```python
from build123d import *

# Parameters (mm, degrees)
SKETCH1_R           = 14
SKETCH1_R_2         = 8
BOSS_EXTRUDE1_DEPTH = 3.5
CUT_EXTRUDE1_START  = -0.5
SKETCH2_R           = 13
SKETCH2_R_2         = 9
CUT_EXTRUDE1_DEPTH  = 22.5


with BuildPart() as part:
    # Sketch1 → Boss-Extrude1 (new, symmetric)
    with BuildSketch(Plane.XY):
        Circle(SKETCH1_R)
        Circle(SKETCH1_R_2, mode=Mode.SUBTRACT)
    extrude(amount=BOSS_EXTRUDE1_DEPTH, both=True)

    # Sketch2 → Cut-Extrude1 (cut)
    with BuildSketch(Plane.XY.offset(3.5).offset(CUT_EXTRUDE1_START)):
        with Locations(Location((0, 0, 0), (0, 0, 180))):
            Circle(SKETCH2_R)
        with Locations(Location((0, 0, 0), (0, 0, 180))):
            Circle(SKETCH2_R_2, mode=Mode.SUBTRACT)
    cut_extrude1 = extrude(amount=CUT_EXTRUDE1_DEPTH, mode=Mode.SUBTRACT)

    # Mirror1: Cut-Extrude1 across plane
    add(cut_extrude1.mirror(Plane.XY), mode=Mode.SUBTRACT)

    # Mirror1 at the second plane: Cut-Extrude1 across plane
    add(cut_extrude1.mirror(Plane(origin=(0, 0, 0), x_dir=(0, 0, 1), z_dir=(1, 0, 0))), mode=Mode.SUBTRACT)


solid = part.part
```
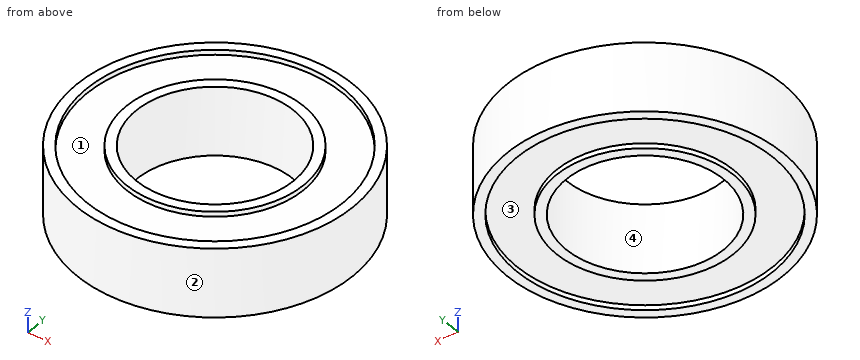
Source: CAD feature listing. Evaluate the final solid. Frame: model axes, mm. Face numbers are marked on the shaded views. A direction names the side the tool comes from. Round coordinates to 2 decimals unless told otherwise and drop trailing zeros. Loops run counter-clockwise (first coordinate to the right, second up) from the corner with the lowest first, then second, coordinate; pieces in that order, holes last.
1. Section query C-C on y = -12.25. Output: boundary loops of the cut face in (x, z), and give its area (3 significant figures).
2. Section query A-A on y = 0. Output: boundary loops of the cut face in (x, z), and give its area (3 significant figures).
3. Section query D-D on z = 1.25. Output: boundary loops of the cut face in (x, y), and give its area (3 significant figures).
4. Mould query, pull axis X, two halves, no side actions, for the marked faces 1 and 2. Classes: released by +X, released by -X, zero draft, split by the parting line, or undercut.
5. Contact query for flat-ended pins moving along their axis: pin 1 (3 mm diameter, centred on y = -8, z = 2, fed in from +X); pin 2 (2 mm diameter, centred on y = -2, z = -1.5, fed in from -X); pin 3 (4 mm diameter, centred on y = 7, z = -2.5, fed in from -X). Output: stop coordinate, or through.
6. Ray query, L1, parallel to Y at x = 0, z = -3.2; L2, parallel to Y at x = 0, z = 1.25; L3, parallel to X at y = -2.75, z = -0.5. Return the intervals inside material, ascending.
7. Access query for the marked faces 3 and 4. Directions: +Z, -Z, +X, -X, +Y, -Y. A direction counts if a zero-diameter tool reaches every point of the face in a straight line with its end or side. Return the directions, or none.
Answers below:
1. outline: (-6.78, -3.5) - (-4.35, -3.5) - (-4.35, -3) - (4.35, -3) - (4.35, -3.5) - (6.78, -3.5) - (6.78, 3.5) - (4.35, 3.5) - (4.35, 3) - (-4.35, 3) - (-4.35, 3.5) - (-6.78, 3.5) - close
1. area: 86.2 mm2
2. outline: (-14, -3.5) - (-13, -3.5) - (-13, -3) - (-9, -3) - (-9, -3.5) - (-8, -3.5) - (-8, 3.5) - (-9, 3.5) - (-9, 3) - (-13, 3) - (-13, 3.5) - (-14, 3.5) - close; (8, -3.5) - (9, -3.5) - (9, -3) - (13, -3) - (13, -3.5) - (14, -3.5) - (14, 3.5) - (13, 3.5) - (13, 3) - (9, 3) - (9, 3.5) - (8, 3.5) - close
2. area: 76.0 mm2
3. outline: circle Ø28 at (0, 0); hole circle Ø16 at (0, 0)
3. area: 415 mm2
4. face 1: undercut
4. face 2: split by the parting line
5. pin 1: stops at x = 12.4
5. pin 2: stops at x = -13.96
5. pin 3: stops at x = -13.08
6. L1: y = -14 to -13, -9 to -8, 8 to 9, 13 to 14
6. L2: y = -14 to -8, 8 to 14
6. L3: x = -13.73 to -7.51, 7.51 to 13.73
7. face 3: -Z
7. face 4: +Z, -Z
